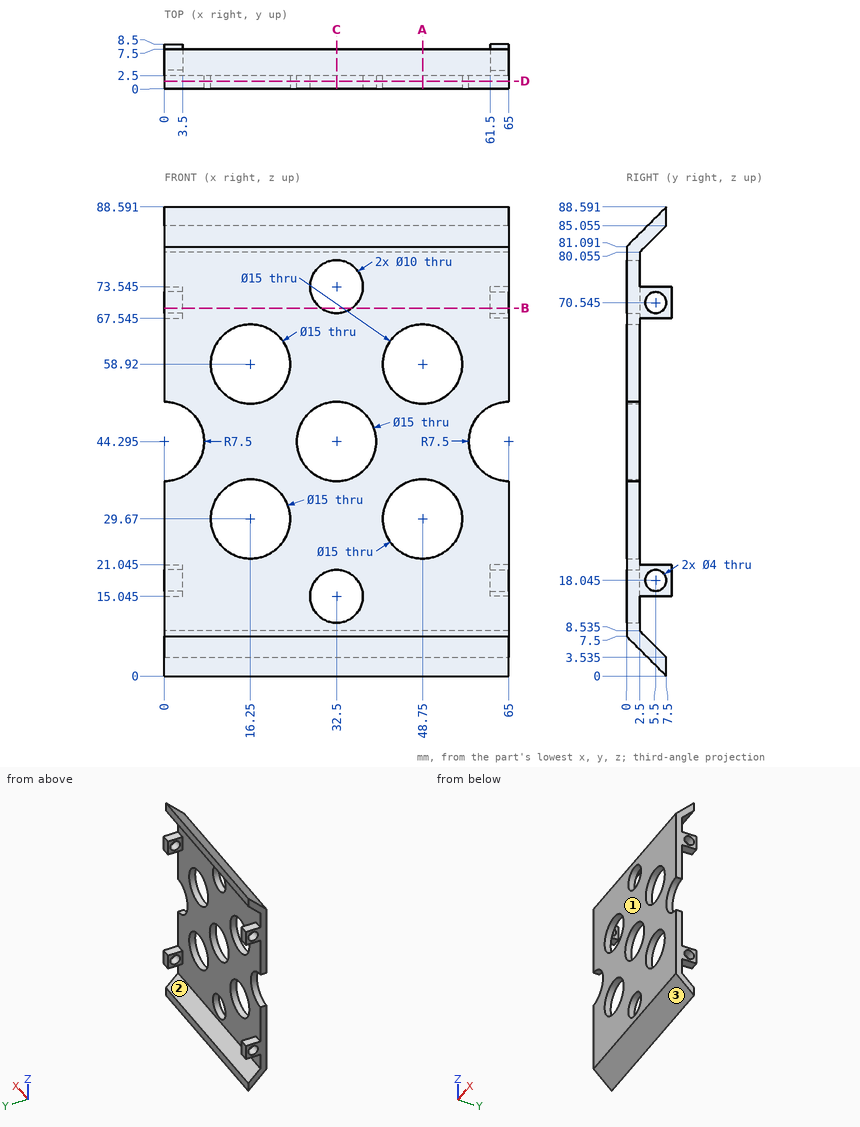
Source: three-view drawing plus pictorial views. Frame: mm from the lowest corner of the part. Give positions to 0.01 mm unless a question says otherwise; leave off trailing zeros. Order: outer loops, then holes, each group sorted by start corner. A loop starts at its lowest first (then second) coordinate and runs counter-clockwise, first axis right, second up. Notation, with made-up numbers: (50, 38.5) - (72, 38.5) arc R21 ccw to (72, 59.5) - close; hole circle Ø10 at (-25, 55). An arc over 180 degrees is marked (long way). Answer as a JSON object with one key per item and string values. Group by question number.
Q1. Cut plane B-B, the plane z = 69.5. Output: boundary loops of the cut face in (x, y) (1 decimal), then the cut area to 3 significant figures.
Q2. Cut plane A-A, the plane x = 48.75. Output: boundary loops of the cut face in (y, z) (1 decimal).
Q3. Cut plane C-C, the plane x = 32.5. Output: boundary loops of the cut face in (y, z) (1 decimal), then the cut area to 3 significant figures.
Q4. First-contact query: pin 1 Ø12 at (x, z) = (16.25, 29.67) entering from -Y; pin 2 Ø1 at (x, y) = (1, 5.5) entering from +Z; pin 3 Ø1 at (x, y) = (62.5, 4) entering from -Z; pin 4 Ø1.8 at (x, z) = (18.5, 1.5) entering from +Y. Flat tips, straight axial feed; report the tip coordinate or a pass-through.
Q5. Line query: probe 1 along Z at (x, y) = (62.8, 5.5) (1 decimal); probe 2 along Z at (x, y) = (48.75, 0.6); probe 3 along X at (y, z) = (0.5, 65) (1 decimal). Output: solid intervals per line, ascending.
Q6. Cut plane D-D, the plane y = 1.5. Count the separate pieces of the cut face and the enclosed holes in it, then the cut area to 3 significant figures.
Q7. Mould query, pull axis Z, two halves, no side actions, for the marked faces 1, 2 and 3. Classes: pulls with the +Z half, pulls with the -Z half, needs draft (parallel to the pull), parting line crosses it, or undercut.
Results:
{
 "1": {"outline": "(0, 0) - (29.6, 0) - (29.6, 2.5) - (3.5, 2.5) - (3.5, 3.8) - (0, 3.8) - close; (0, 7.2) - (3.5, 7.2) - (3.5, 8.5) - (0, 8.5) - close; (35.4, 0) - (65, 0) - (65, 3.8) - (61.5, 3.8) - (61.5, 2.5) - (35.4, 2.5) - close; (61.5, 7.2) - (65, 7.2) - (65, 8.5) - (61.5, 8.5) - close", "area": "166 mm^2"},
 "2": {"outline": "(0, 7.5) - (7.5, 0) - (7.5, 3.5) - (2.5, 8.5) - (2.5, 22.2) - (0, 22.2) - close; (0, 37.2) - (2.5, 37.2) - (2.5, 51.4) - (0, 51.4) - close; (0, 66.4) - (2.5, 66.4) - (2.5, 80.1) - (7.5, 85.1) - (7.5, 88.6) - (0, 81.1) - close"},
 "3": {"outline": "(0, 7.5) - (7.5, 0) - (7.5, 3.5) - (2.5, 8.5) - (2.5, 10) - (0, 10) - close; (0, 20) - (2.5, 20) - (2.5, 36.8) - (0, 36.8) - close; (0, 51.8) - (2.5, 51.8) - (2.5, 68.5) - (0, 68.5) - close; (0, 78.5) - (2.5, 78.5) - (2.5, 80.1) - (7.5, 85.1) - (7.5, 88.6) - (0, 81.1) - close", "area": "138 mm^2"},
 "4": {"pin 1": "through", "pin 2": "z = 87.09", "pin 3": "z = 3", "pin 4": "y = 7.5"},
 "5": {"probe 1": "2 to 5.5, 15 to 16, 20 to 21, 67.5 to 68.5, 72.5 to 73.5, 83.1 to 86.6", "probe 2": "6.9 to 22.17, 37.17 to 51.42, 66.42 to 81.69", "probe 3": "0 to 11.9, 20.6 to 44.4, 53.1 to 65"},
 "6": {"separate pieces": "1", "enclosed holes": "7", "area": "3,760 mm^2"},
 "7": {"face 1": "needs draft", "face 2": "undercut", "face 3": "pulls with the -Z half"}
}
